Part model, mm, in its own coordinate system. A direction names the side the tool comes from. Coordinates: 2 decimals unless noted, no trailing zeros. Order: outer loops, then holes, each group sorted by start corner. A loop starts at its lowest first (then second) coordinate and runs counter-clockwise, first axis right, second up.
1) Cut at C-C (z = 7). List the corners of the cut face in (x, y), and give its area (3 significant figures).
2) Cut at A-A (x = 0). List the corners of the cut face in (y, z).
3) Tool access for faces 1 (the flat face through (0, 119, 0.5)), 2 (the flat face through (0, 150, 10)), 3 (the flat face through (0, 119, 0)): list every direction of +Z, -Z, +X, -X, +Y, -Y with a clear straight run to the whole face (end or side of a thin tool).
4) Cut at B-B (y = 119.5). List the corners of the cut face in (x, z), and give its area (3 significant figures).
5) Pin check, flat tips, straight feed: pin 1 Ø8 at (x, y) = (-1, 155.5) entering from -Z; pin 2 Ø2.5 at (x, z) = (1, 6.5) entering from +Y; pin 3 Ø2.5 at (x, y) = (-0.5, 119) entering from +Z. Stop position of each tip, or through.
6) Wall check: L1, parallel to Y at x = 0, z = 0.35; L2, parallel to Y at x = 2.25, z = 6.5; L3, parallel to Z at x = 13, y = 154. Give the ranges that are in metal, low to high.
7) Mould opens along X. For faces 4 (the flat face through (0, 129.548, 5)), 5 (the flat face through (3.937, 123.8, 0.2)), 6 (the cylindrical face through (-0.2, 125.19, 0.25)) say: +X half, -X half, draft (parallel to the pull), parting line (faces both ways), or undercut.
```python
from build123d import *

# Parameters (mm, degrees)
SKETCH1_W           = 7.874
SKETCH1_H           = 22.225
SKETCH1_R           = 1.504480346
BOSS_EXTRUDE1_DEPTH = 0.5
SKETCH2_W           = 7.874
SKETCH2_H           = 0.5
BOSS_EXTRUDE2_DEPTH = 10
SKETCH3_W           = 30
SKETCH3_H           = 0.5
BOSS_EXTRUDE3_DEPTH = 40


with BuildPart() as part:
    # Sketch1 → Boss-Extrude1 (new body)
    with BuildSketch(Plane.XY):
        with Locations((0, 118.9355)):
            Rectangle(SKETCH1_W, SKETCH1_H)
        with Locations((0, 123.698)):
            Circle(SKETCH1_R, mode=Mode.SUBTRACT)
        with Locations((0, 110.998)):
            Circle(SKETCH1_R, mode=Mode.SUBTRACT)
    extrude(amount=BOSS_EXTRUDE1_DEPTH)

    # Sketch2 → Boss-Extrude2 (add)
    with BuildSketch(Plane.XY.offset(0.5)):
        with Locations((0, 129.798)):
            Rectangle(SKETCH2_W, SKETCH2_H)
    extrude(amount=BOSS_EXTRUDE2_DEPTH)

    # Sketch3 → Boss-Extrude3 (add)
    with BuildSketch(Plane(origin=(0, 130.048, 0), x_dir=(1, 0, 0), z_dir=(0, 1, 0))):
        with Locations((0, -10.25)):
            Rectangle(SKETCH3_W, SKETCH3_H)
    extrude(amount=BOSS_EXTRUDE3_DEPTH)


solid = part.part
```
Geometry check:
1. outline: (-3.94, 129.55) - (3.94, 129.55) - (3.94, 130.05) - (-3.94, 130.05) - close
1. area: 3.94 mm2
2. outline: (107.82, 0) - (109.49, 0) - (109.49, 0.5) - (107.82, 0.5) - close; (112.5, 0) - (122.19, 0) - (122.19, 0.5) - (112.5, 0.5) - close; (125.2, 0) - (130.05, 0) - (130.05, 10) - (170.05, 10) - (170.05, 10.5) - (129.55, 10.5) - (129.55, 0.5) - (125.2, 0.5) - close
3. face 1: +Z, +X, -X, -Y
3. face 2: -Z, +X, -X, +Y
3. face 3: -Z, +X, -X, +Y, -Y
4. outline: (-3.94, 0) - (3.94, 0) - (3.94, 0.5) - (-3.94, 0.5) - close
4. area: 3.94 mm2
5. pin 1: stops at z = 10
5. pin 2: stops at y = 130.05
5. pin 3: stops at z = 0.5
6. L1: y = 107.82 to 109.49, 112.5 to 122.19, 125.2 to 130.05
6. L2: y = 129.55 to 130.05
6. L3: z = 10 to 10.5
7. face 4: draft
7. face 5: +X half
7. face 6: undercut
